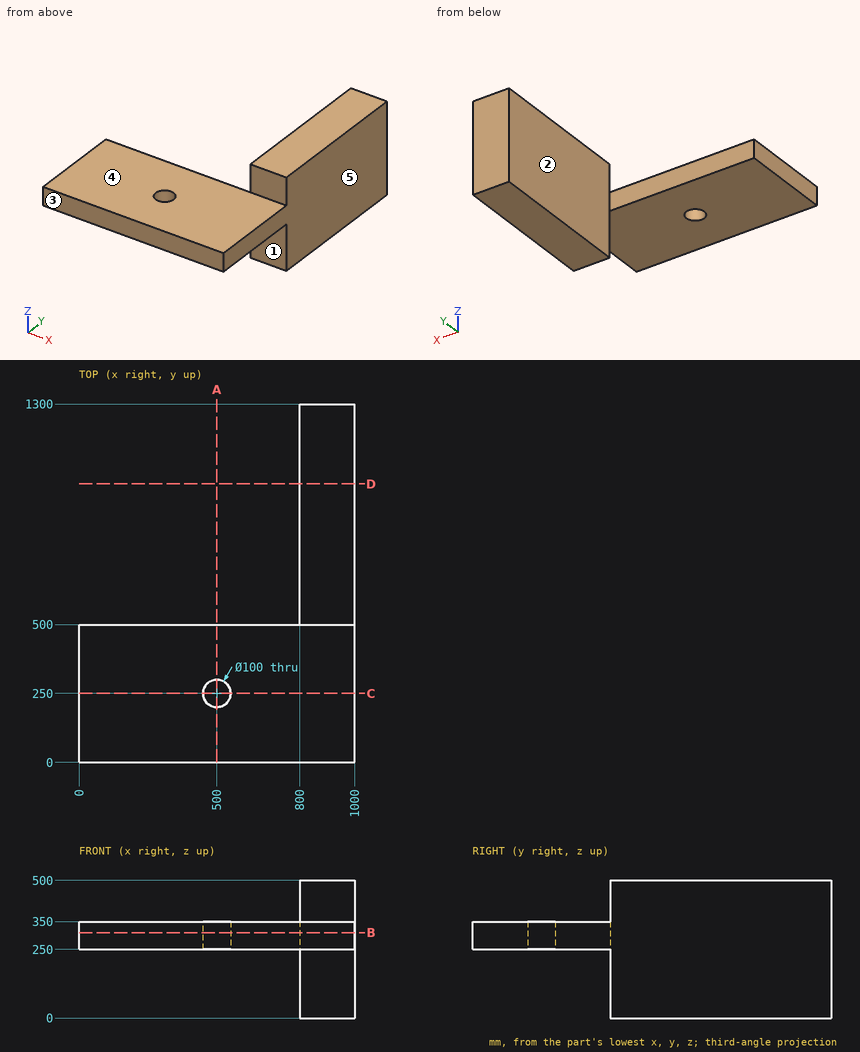
Can you work these out from the drawing? Everything is in mm from the part's minimum corner. A direction names the side the tool comes from. Round coordinates to 2 decimals unless told otherwise and drop trailing zeros. Order: outer loops, then holes, each group sorted by start corner. A loop starts at its lowest first (then second) coordinate and runs counter-clockwise, first axis right, second up. Notation, with made-up numbers: (9.5, 23.5) -> (64.5, 23.5) arc R13 ccw to (64.5, 43.5) -> close; hole circle Ø2 at (16, 88.5). An arc over 180 degrees is marked (long way). Return JSON: item names as keys, results as strings. Group by question number.
1. Will these pins go through, and if not, where does the flat tip stop? pin 1 (6 mm diameter, centred on x = 635.5, y = 159, fed in from -Z); pin 2 (1.5 mm diameter, centred on x = 785, y = 208, fed in from +Z).
2. I need wall thicknesses on line 1 (Y direction, x = 500, z = 302); line 2 (X direction, y = 250, z = 285.5); line 3 (X direction, y = 1092, z = 330). Which ranges of each line are inside material? Lowest first, please. Write a range as [from, to].
3. If we section it at A-A, the plane x = 500: Write out the boundary of the cut face in (y, z).
4. Which directions (+Z, -Z, +X, -X, +Y, -Y) give clear straight access to the entire face, cutting with the end or side of a thin tool? Please do the marked faces 1, 2, 3, 4 and 5.
5. If we section it at C-C, the plane y = 250: Write out the boundary of the cut face in (x, z).
6. If we section it at B-B, the plane z = 310: Write out the boundary of the cut face in (x, y).
7. If we section it at D-D, the plane y = 1010: Write out the boundary of the cut face in (x, z), then the cut area to 3 significant figures.
Output values:
{
 "1": {"pin 1": "z = 250", "pin 2": "z = 350"},
 "2": {"line 1": "[0, 200], [300, 500]", "line 2": "[0, 450], [550, 1000]", "line 3": "[800, 1000]"},
 "3": {"outline": "(0, 250) -> (200, 250) -> (200, 350) -> (0, 350) -> close; (300, 250) -> (500, 250) -> (500, 350) -> (300, 350) -> close"},
 "4": {"face 1": "-Z, +X, -X, -Y", "face 2": "+Z, -Z, -X, +Y", "face 3": "+Z, -Z, +X, -X, -Y", "face 4": "+Z, +X, -X, -Y", "face 5": "+Z, -Z, +X, +Y, -Y"},
 "5": {"outline": "(0, 250) -> (450, 250) -> (450, 350) -> (0, 350) -> close; (550, 250) -> (1000, 250) -> (1000, 350) -> (550, 350) -> close"},
 "6": {"outline": "(0, 0) -> (1000, 0) -> (1000, 1300) -> (800, 1300) -> (800, 500) -> (0, 500) -> close; hole circle Ø100 at (500, 250)"},
 "7": {"outline": "(800, 0) -> (1000, 0) -> (1000, 500) -> (800, 500) -> close", "area": "100,000 mm²"}
}
